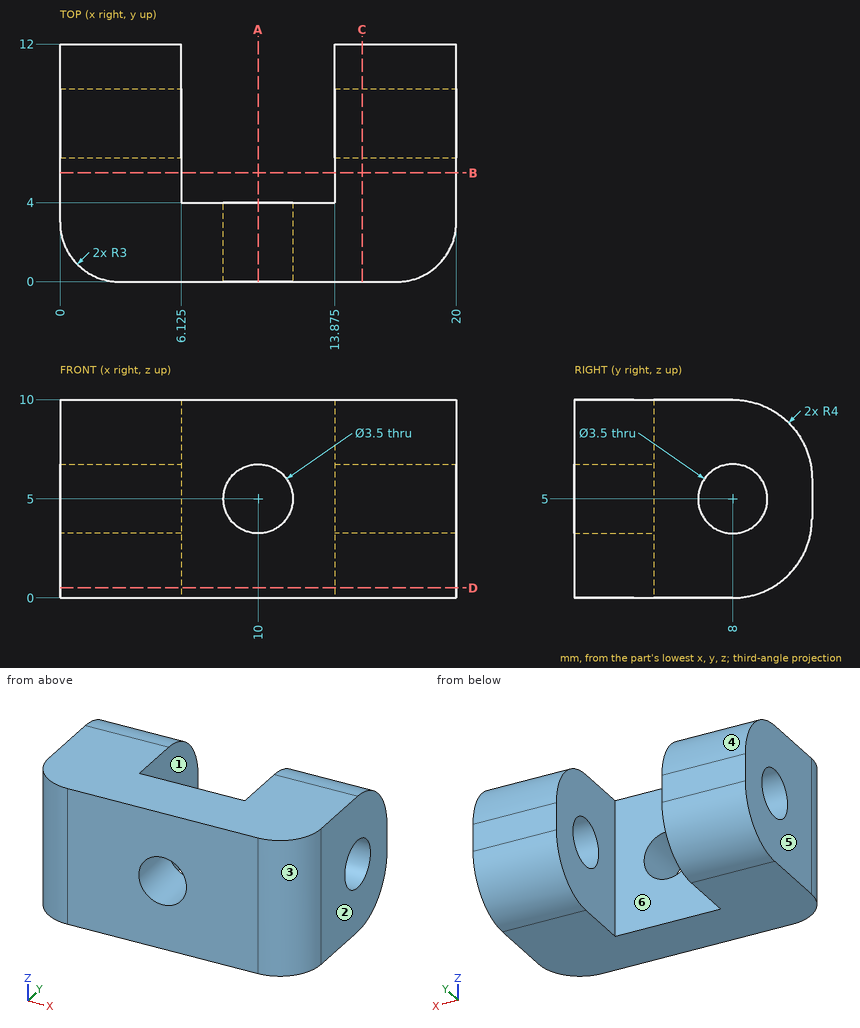
Input: dimensioned drawing with shaded views. Units: mm. Origin: part minimum x, y, z. A direction names the side the tool comes from. Round coordinates to 2 decimals unless told otherwise and drop trailing zeros. Order: outer loops, then holes, each group sorted by start corner. A loop starts at its lowest first (then second) coordinate and runs counter-clockwise, first axis right, second up.
Q1. Section C-C, the plane x = 15.25. Output: boundary loops of the cut face in (y, z).
Result sheet:
outline: (0, 0) - (8, 0) arc R4 ccw to (12, 4) - (12, 6) arc R4 ccw to (8, 10) - (0, 10) - close; hole circle Ø3.5 at (8, 5)
Q2. Access query for the marked faces 1 and 2. Directions: +Z, -Z, +X, -X, +Y, -Y. A direction counts if a zero-diameter tool reaches every point of the face in a straight line with its end or side. Return the directions, or none.
Result sheet:
face 1: +Z, -Z, +Y
face 2: +Z, -Z, +X, +Y, -Y
Q3. Pin query (flat end, axial travel): pin 1 (2 mm diameter, centred on y = 8, z = 5, fed in from +X); pin 2 (2.5 mm diameter, centred on y = 7, z = 6, fed in from +X); pin 3 (4 mm diameter, centred on x = 8.5, z = 6, fed in from +Y). Return the tip coordinate at first contact, or that it passes through.
Result sheet:
pin 1: passes through
pin 2: stops at x = 20
pin 3: stops at y = 4
Q4. Material intervals for probe 1 along Z at (x, y) = (10, 2.05); probe 2 along X at (y, z) = (5.5, 9.5) (3 decimals); probe 3 along Y at (x, z) = (5, 5), sorted ascending.
Result sheet:
probe 1: z = 0 to 3.25, 6.75 to 10
probe 2: x = 0 to 6.125, 13.875 to 20
probe 3: y = 0 to 6.25, 9.75 to 12
Q5. Section A-A, the plane x = 10. Output: boundary loops of the cut face in (y, z), and give its area (3 significant figures).
Result sheet:
outline: (0, 0) - (4, 0) - (4, 3.25) - (0, 3.25) - close; (0, 6.75) - (4, 6.75) - (4, 10) - (0, 10) - close
area: 26.0 mm2
Q6. Mould query, pull axis X, two halves, no side actions, for the marked faces 3, 4, 5 and 6. Classes: released by +X, released by -X, zero draft, split by the parting line, or undercut.
Result sheet:
face 3: released by +X
face 4: zero draft
face 5: released by -X
face 6: undercut
Q7. Section B-B, the plane y = 5.5. Output: boundary loops of the cut face in (x, z) (3 decimals).
Result sheet:
outline: (0, 0) - (6.125, 0) - (6.125, 10) - (0, 10) - close; (13.875, 0) - (20, 0) - (20, 10) - (13.875, 10) - close
Q8. Section D-D, the plane z = 0.5. Output: boundary loops of the cut face in (x, y) (1 decimal).
Result sheet:
outline: (0, 3) arc R3 ccw to (3, 0) - (17, 0) arc R3 ccw to (20, 3) - (20, 9.9) - (13.9, 9.9) - (13.9, 4) - (6.1, 4) - (6.1, 9.9) - (0, 9.9) - close
